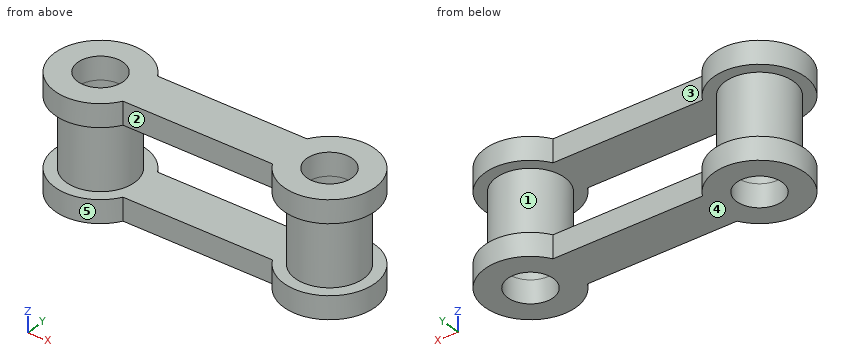
```python
from build123d import *
from build123d.topology import SkipClean

# Parameters (mm, degrees)
SKETCH_1_R      = 2
EXTRUDE_1_DEPTH = 2
EXTRUDE_START   = 6
SKETCH_2_R      = 3
SKETCH_2_R_2    = 2
EXTRUDE_2_DEPTH = 6


with BuildPart() as part:
    # 草图1 → 凸台-拉伸1 (new body)
    with BuildSketch(Plane.XY):
        with BuildLine():
            Line((-0.652657961, 3.769166536), (12.40050126, 3.769166536))
            ThreePointArc((12.40050126, 3.769166536), (19.873921649, 1.785394675), (12.40050126, -0.198377186))
            Line((12.40050126, -0.198377186), (-0.652657961, -0.198377186))
            ThreePointArc((-0.652657961, -0.198377186), (-8.126078351, 1.785394675), (-0.652657961, 3.769166536))
        make_face()
        with Locations((-4.126078351, 1.785394675)):
            Circle(SKETCH_1_R, mode=Mode.SUBTRACT)
        with Locations(Location((15.873921649, 1.785394675, 0), (0, 0, 180))):
            Circle(SKETCH_1_R, mode=Mode.SUBTRACT)
    extrude_1 = extrude(amount=EXTRUDE_1_DEPTH)

    # 草图2 → 凸台-拉伸2 (add)
    # profile 1 of 2: a face of its own
    with SkipClean():  # the faces are left unmerged after this step: merging them gives an invalid solid
        with BuildSketch(Plane(origin=(0, 0, 0), x_dir=(-1, 0, 0), z_dir=(0, 0, -1)).offset(EXTRUDE_START)):
            with Locations(Location((-15.873921649, 1.785394675, 0), (0, 0, 180))):
                Circle(SKETCH_2_R)
            with Locations((-15.873921649, 1.785394675)):
                Circle(SKETCH_2_R_2, mode=Mode.SUBTRACT)
        # profile 2 of 2: a face of its own
        with BuildSketch(Plane(origin=(0, 0, 0), x_dir=(-1, 0, 0), z_dir=(0, 0, -1)).offset(EXTRUDE_START)):
            with Locations(Location((4.126078351, 1.785394675, 0), (0, 0, 180))):
                Circle(SKETCH_2_R)
            with Locations((4.126078351, 1.785394675)):
                Circle(SKETCH_2_R_2, mode=Mode.SUBTRACT)
        extrude(amount=-EXTRUDE_2_DEPTH)

    # 镜向1: 凸台-拉伸1 across plane
    with SkipClean():  # the faces are left unmerged after this step: merging them gives an invalid solid
        add(extrude_1.mirror(Plane(origin=(0, 0, -3), x_dir=(1, 0, 0), z_dir=(0, 0, -1))))


solid = part.part
```
Work out the finished part from the listing and answer in its coordinate system (mm). Face numbers are marked on the shaded views. A direction names the side the tool comes from. Give positions to 0.01 mm unless a question says otherwise; leave off trailing zeros. Loops run counter-clockwise (first coordinate to the right, second up) from the corner with the lowest first, then second, coordinate; pieces in that order, holes last. Notation, with made-up numbers: (-15, 3.5) -> (20, 3.5) arc R16 ccw to (20, 19.5) -> close; hole circle Ø10 at (71.5, 89.5). An arc over 180 degrees is marked (long way). One line per question, with ' | ' between items. Start each with the question number.
1) Section C-C, the plane y = -1.5 is taken. Determine the outline of the cut face in (x, z), then the cut area to 3 significant figures.
2) Each of these flat-tipped pins is pushed along its axis until it touches: pin 1 (1.6 mm diameter, centred on x = 6, z = 1.5, fed in from +Y); pin 2 (1 mm diameter, centred on x = 8.5, z = 1.5, fed in from -Y); pin 3 (3 mm diameter, centred on y = 4.5, z = -0.5, fed in from +X). Where does it stop, or does it pass through?
3) Section B-B, the plane x = 9.25 is taken. Determine the outline of the cut face in (y, z).
4) Section D-D, the plane z = -7 is taken. Determine the outline of the cut face in (x, y).
5) Determine the mould class of the marked faces 4 and 5 for opening direction X: +X half, -X half, draft (parallel to the pull), parting line (faces both ways), or undercut.
6) Straight lines are drawn through the part: L1, parallel to X at y = 1.75, z = 1; L2, parallel to X at y = 1.75, z = -1; L3, parallel to X at y = 2.75, z = -6.25. For each, find the intervals that lie inside material, in ascending order.
7) Section A-A, the plane y = 2.25 is taken. Determine the outline of the cut face in (x, z), then the cut area to 3 significant figures.
8) For the marked faces 1, 2 and 3, determine the directions among +Z, -Z, +X, -X, +Y, -Y from which every point of the face is accessible in a straight line to the end or side of a thin tool.
Resolved:
1) outline: (-6.41, -8) -> (-1.84, -8) -> (-1.84, -6) -> (-6.41, -6) -> close; (-6.41, 0) -> (-1.84, 0) -> (-1.84, 2) -> (-6.41, 2) -> close; (13.59, -8) -> (18.16, -8) -> (18.16, -6) -> (13.59, -6) -> close; (13.59, 0) -> (18.16, 0) -> (18.16, 2) -> (13.59, 2) -> close | area: 36.5 mm2
2) pin 1: y = 3.77 | pin 2: y = -0.2 | pin 3: x = 19.66
3) outline: (-0.2, -8) -> (3.77, -8) -> (3.77, -6) -> (-0.2, -6) -> close; (-0.2, 0) -> (3.77, 0) -> (3.77, 2) -> (-0.2, 2) -> close
4) outline: (-0.65, -0.2) -> (12.4, -0.2) arc R4 ccw (long way) to (12.4, 3.77) -> (-0.65, 3.77) arc R4 ccw (long way) to start; hole circle Ø4 at (-4.13, 1.79); hole circle Ø4 at (15.87, 1.79)
5) face 4: draft | face 5: undercut
6) L1: -8.13 to -6.13, -2.13 to 13.87, 17.87 to 19.87 | L2: -7.13 to -6.13, -2.13 to -1.13, 12.87 to 13.87, 17.87 to 18.87 | L3: -8.01 to -5.88, -2.37 to 14.12, 17.63 to 19.76
7) outline: (-8.1, -8) -> (-6.07, -8) -> (-6.07, 2) -> (-8.1, 2) -> (-8.1, 0) -> (-7.09, 0) -> (-7.09, -6) -> (-8.1, -6) -> close; (-2.18, -8) -> (13.93, -8) -> (13.93, 2) -> (-2.18, 2) -> close; (17.82, -8) -> (19.85, -8) -> (19.85, -6) -> (18.84, -6) -> (18.84, 0) -> (19.85, 0) -> (19.85, 2) -> (17.82, 2) -> close; hole (-1.16, -6) -> (12.91, -6) -> (12.91, 0) -> (-1.16, 0) -> close | area: 105 mm2
8) face 1: none | face 2: +Z, -Z, -Y | face 3: +Z, -Z, +Y
